For this review, take the finished solid that the model builds, in its own axes (mm). Face numbers are marked on the shaded views. Coordinates: 2 decimals unless noted, no trailing zeros. Order: outer loops, then holes, each group sorted by start corner. A loop starts at its lowest first (then second) coordinate and runs counter-clockwise, first axis right, second up. Notation, with made-up numbers: M 77.5,46 L 112.5,46 A22 cw 112.5,68 Z; hole C 84.25,67.5 d2. An arc over 180 degrees is marked long. Use CSV: the item, a comma, the result in double quotes.
```python
from build123d import *

# Parameters (mm, degrees)
SKETCH1_W           = 230
SKETCH1_H           = 160
BOSS_EXTRUDE1_DEPTH = 0.5
BOSS_EXTRUDE2_DEPTH = 0.5


with BuildPart() as part:
    # Sketch1 → Boss-Extrude1 (new body)
    with BuildSketch(Plane(origin=(0, 0, 0), x_dir=(1, 0, 0), z_dir=(0, 1, 0))):
        Rectangle(SKETCH1_W, SKETCH1_H)
    extrude(amount=BOSS_EXTRUDE1_DEPTH)

    # Sketch2 → Boss-Extrude2 (add)
    with BuildSketch(Plane(origin=(0, 0.5, 0), x_dir=(1, 0, 0), z_dir=(0, 1, 0))):
        with BuildLine():
            Line((-97.32233047, 63.029437252), (-98.736544033, 63.029437252))
            Line((-98.736544033, 63.029437252), (-105, 63.029437252))
            ThreePointArc((-105, 63.029437252), (-112.071067812, 60.100505063), (-115, 53.029437252))
            Line((-115, 53.029437252), (-115, -80))
            Line((-115, -80), (115, -80))
            Line((115, -80), (115, 53.029437252))
            ThreePointArc((115, 53.029437252), (112.071067812, 60.100505063), (105, 63.029437252))
            Line((105, 63.029437252), (98.736544033, 63.029437252))
            Line((98.736544033, 63.029437252), (97.32233047, 63.029437252))
            Line((97.32233047, 63.029437252), (-97.32233047, 63.029437252))
        make_face()
        with BuildLine():
            Line((-105, 62.029437252), (105, 62.029437252))
            ThreePointArc((105, 62.029437252), (111.363961031, 59.393398282), (114, 53.029437252))
            Line((114, 53.029437252), (114, -79))
            Line((114, -79), (-114, -79))
            Line((-114, -79), (-114, 53.029437252))
            ThreePointArc((-114, 53.029437252), (-111.363961031, 59.393398282), (-105, 62.029437252))
        make_face(mode=Mode.SUBTRACT)
        Polygon((-115, 80), (-115, 79.292893219), (-98.736544033, 63.029437252), (-97.32233047, 63.029437252), (-114.292893219, 80), align=None)
        Polygon((114.292893219, 80), (97.32233047, 63.029437252), (98.736544033, 63.029437252), (115, 79.292893219), (115, 80), align=None)
    extrude(amount=BOSS_EXTRUDE2_DEPTH)


solid = part.part
```
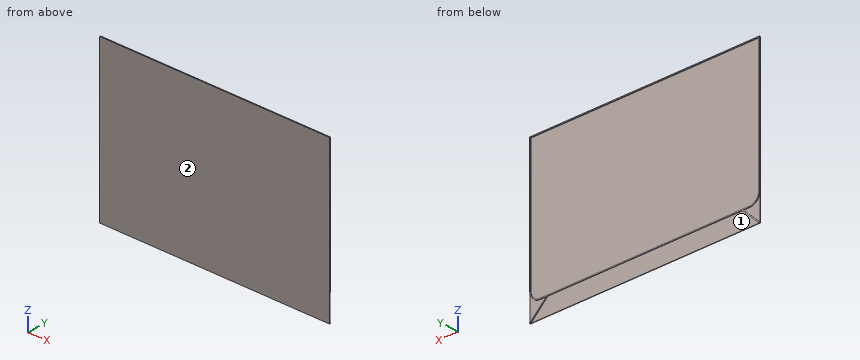
Item 1: Add section B-B on z = 61. State the section outline as (x, y) points, and give its area (3 significant figures).
Solutions:
outline,"M -115,0 L 115,0 L 115,1 L 114,1 L 114,0.5 L -114,0.5 L -114,1 L -115,1 Z"
area,"116 mm^2"
Item 2: Add section A-A on y = 0.7. State the section outline as (x, z) points.
Solutions:
outline,"M -115,-80 L -114.29,-80 L -97.32,-63.03 L 97.32,-63.03 L 114.29,-80 L 115,-80 L 115,-79.29 L 98.74,-63.03 L 105,-63.03 A10 ccw 115,-53.03 L 115,80 L -115,80 L -115,-53.03 A10 ccw -105,-63.03 L -98.74,-63.03 L -115,-79.29 Z; hole M -114,-53.03 A9 ccw -105,-62.03 L 105,-62.03 A9 ccw 114,-53.03 L 114,79 L -114,79 Z"
Item 3: Add section D-D on z = -55.5. State the section outline as (x, y) points, and give its area (3 significant figures).
Solutions:
outline,"M -115,0 L 115,0 L 115,0.5 L 114.69,0.5 L 114.69,1 L 113.65,1 L 113.65,0.5 L -113.65,0.5 L -113.65,1 L -114.69,1 L -114.69,0.5 L -115,0.5 Z"
area,"116 mm^2"
Item 4: Draft analysis for pull direction X (two halves, no side actions). For the marked faces 1 and 2, state which applies: released by +X, released by -X, zero draft, split by the parting line, or undercut.
Solutions:
face 1,"undercut"
face 2,"zero draft"
Item 5: Add section C-C on x = -79.5. State the section outline as (y, z) points, and give its area (3 significant figures).
Solutions:
outline,"M 0,-80 L 0.5,-80 L 0.5,-63.03 L 1,-63.03 L 1,-62.03 L 0.5,-62.03 L 0.5,79 L 1,79 L 1,80 L 0,80 Z"
area,"81.0 mm^2"
Item 6: To check wall thickness, follow line 1 along X through (y, z) = (0.75, -15.5); line 2 along Z through (x, y) = (82.5, 0.8); line 3 along Z through (x, y) = (103.5, 0.9). State the ranges of each line that lie inside material, in increasing order. Write a range as [from, to].
Solutions:
line 1,"[-115, -114], [114, 115]"
line 2,"[-63.03, -62.03], [79, 80]"
line 3,"[-69.21, -67.79], [-63.03, -62.03], [79, 80]"
Item 7: Clearance check with a flat-ended pin moving along its axis: pin 1 Ø12 at (x, z) = (82.5, -7.5) entering from +Y. State where the tip first meets the part, or that it passes through.
Solutions:
pin 1,"y = 0.5"
